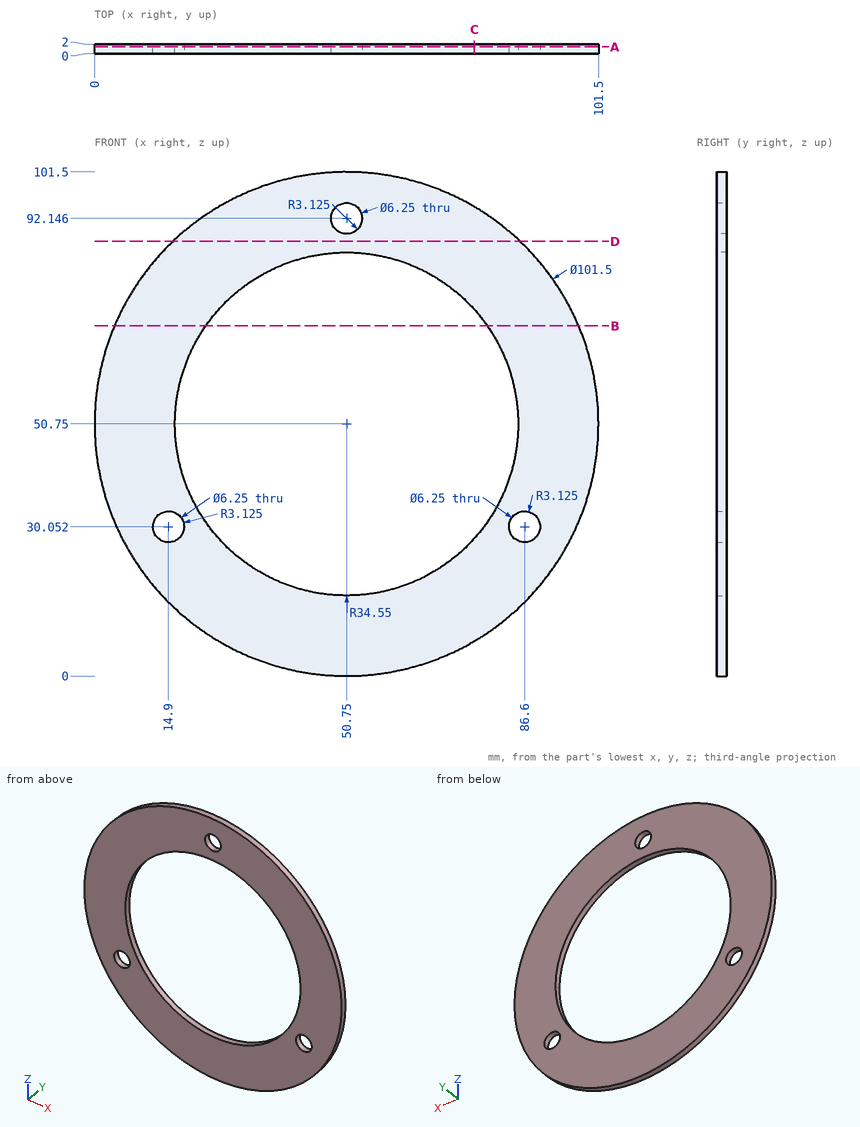
Could you check a few things on this drawing? It's one solid part, dimensions in mm from its lowest x, y, z. Round coordinates to 2 decimals unless told otherwise and drop trailing zeros. Write each loop counter-clockwise with the first axis right and the second up, starting at its lowest first coordinate (ties: lowest second). Pieces come first, ordered by that corner, then holes.
Q1. If we section it at C-C on x = 76.5: Write out the boundary of the cut face in (y, z), plus the area to 3 significant figures.
Q2. If we section it at A-A on y = 1.4: Give the number of separate pieces and of enclosed holes in the cut face, plus the area to 3 significant figures.
Q3. If we section it at B-B on z = 70.5: Write out the boundary of the cut face in (x, y).
Q4. Please list where these lines run through material, in increasing order: probe 1 along X at (y, z) = (0.3, 31.5); probe 2 along Z at (x, y) = (14, 0.2); probe 3 along Z at (x, y) = (14.9, 1.6).
Q5. Will these pins go through, and if not, where does the flat tip stop? P1, Ø1, axis at y = 1.5, z = 62, coming from the -X side; P2, Ø2, axis at x = 86.5, z = 86.5, coming from the -Y side.
Q6. If we section it at D-D on z = 87.5: Write out the boundary of the cut face in (x, y), plus the area to 3 significant figures.
Answer below:
1. outline: (0, 7.02) - (2, 7.02) - (2, 27.71) - (0, 27.71) - close; (0, 73.79) - (2, 73.79) - (2, 94.48) - (0, 94.48) - close
1. area: 82.8 mm2
2. separate pieces: 1
2. enclosed holes: 4
2. area: 4,250 mm2
3. outline: (4, 0) - (22.4, 0) - (22.4, 2) - (4, 2) - close; (79.1, 0) - (97.5, 0) - (97.5, 2) - (79.1, 2) - close
4. probe 1: x = 3.79 to 12.13, 17.67 to 22.06, 79.44 to 83.83, 89.37 to 97.71
4. probe 2: z = 15.75 to 27.06, 33.04 to 85.75
4. probe 3: z = 14.83 to 26.93, 33.18 to 86.67
5. P1: stops at x = 1.15
5. P2: stops at y = 0
6. outline: (15.75, 0) - (85.75, 0) - (85.75, 2) - (15.75, 2) - close
6. area: 140 mm2
